Check sheet for the modelled part. Datum: model origin and axes. Units: mm. Coordinates: 2 decimals unless noted, no trailing zeros. Order: outer loops, then holes, each group sorted by start corner. A loop starts at its lowest first (then second) coordinate and runs counter-clockwise, first axis right, second up. Notation, with made-up numbers: (50, -35.5) -> (57, -35.5) arc R33 ccw to (57, -0.5) -> close; hole circle Ø1 at (79, 14). An arc over 180 degrees is marked (long way). Put each result on its own line as item: value. Start each with the question number.
```python
from build123d import *

# Parameters (mm, degrees)
F0_W      = 80
F0_H      = 120
F0_R      = 9.75
F0_R_2    = 4.25
F1_DEPTH  = 4
F3_W      = 80
F3_H      = 20
F4_DEPTH  = 10
F5_W      = 6
F5_H      = 6
F5_R      = 0.95
F6_DEPTH  = 10
F7_R      = 2.99999
F11_W     = 97.9346781969
F11_H     = 127.8536170721
F11_W_2   = 72.8027671576
F11_H_2   = 72.8027634323
F12_DEPTH = 10


# Not quite as in the source:
# - a fillet or chamfer is up to 0.001 mm smaller than in the source, because OpenCascade refuses the exact size


with BuildPart() as f1:
    # F0 (on Front) → F1 (new body)
    with BuildSketch(Plane.XZ):
        Rectangle(F0_W, F0_H)
        with Locations((0, -24.624)):
            Circle(F0_R, mode=Mode.SUBTRACT)
        with Locations((-24.032204955, 17.001)):
            Circle(F0_R, mode=Mode.SUBTRACT)
        with Locations((0, 3.126)):
            Circle(F0_R, mode=Mode.SUBTRACT)
        with Locations((0, 29.876)):
            Circle(F0_R_2, mode=Mode.SUBTRACT)
        with Locations((24.032204955, 17.001)):
            Circle(F0_R, mode=Mode.SUBTRACT)
    extrude(amount=F1_DEPTH)

    # F3 (on face) → F4 (cut)
    with BuildSketch(Plane.XZ.offset(4)):
        with Locations((0, -50)):
            Rectangle(F3_W, F3_H)
    extrude(amount=-F4_DEPTH, mode=Mode.SUBTRACT)

    # F8: F6 across plane


with BuildPart() as f6:
    # F5 (on face) → F6 (new body)
    with BuildSketch(Plane.XZ.offset(4)):
        with Locations((43, 3)):
            Rectangle(F5_W, F5_H)
        with Locations((42.5, 3.126)):
            Circle(F5_R, mode=Mode.SUBTRACT)
    extrude(amount=-F6_DEPTH)

    # F7 (radius 3 in the source; OpenCascade refuses exactly that, so slightly less here)
    f7_edges = [f6.edges().sort_by_distance(p)[0] for p in [
        (46, 1, 0),
        (46, 1, 6),
    ]]
    fillet(f7_edges, radius=F7_R)


with BuildPart() as f1_1:
    add(f1.part)
    add(f6.part.mirror(Plane.YZ))


with BuildPart() as f12_tool:
    # F11 (on face) → F12 (new body)
    with BuildSketch(Plane.XZ.offset(4)):
        with Locations((1.1506490409, -1.4746189117)):
            Rectangle(F11_W, F11_H)
        with Locations((0.1533515751, -0.2778600901)):
            Rectangle(F11_W_2, F11_H_2, mode=Mode.SUBTRACT)
    extrude(amount=-F12_DEPTH)


with BuildPart() as f1_2:
    add(f1_1.part)

    # F12: cut by f12_tool
    add(f12_tool.part, mode=Mode.SUBTRACT)


with BuildPart() as f6_1:
    add(f6.part)

    # F12: cut by f12_tool
    add(f12_tool.part, mode=Mode.SUBTRACT)


solid = f1_2.part
```
1) Sectioned sample at A-A (x = -28.5). Record the boundary of the cut face in (y, z), plus the area to 3 significant figures.
2) Sectioned sample at D-D (z = 10). Record the boundary of the cut face in (x, y).
3) Sectioned sample at B-B (x = 0). Record the boundary of the cut face in (y, z), plus the area to 3 significant figures.
4) Scan lines: line 1 along X through (y, z) = (-1.6, 14); line 2 along Z through (x, y) = (-5.5, -2.6); line 3 along X through (y, z) = (-2.25, 21). Record each from-to range of solid material in increasing order. Write a range as [from, to].
5) Mould release check, pull along Z, two halves, no side actions. Record for faces 1 (the flat face through (0, -2, 36.124)), 2 (the flat face through (0, -2, -36.679)), 3 (the cylindrical face through (-7.737, -1.972, -2.807)), 4 (the flat face through (1, -4, -8)): +Z half, -Z half, draft (parallel to the pull), parting line (faces both ways), or undercut.
6) Sectioned sample at C-C (y = -2.9). Record the boundary of the cut face in (x, z).
Entries:
1. outline: (-4, -36.68) -> (0, -36.68) -> (0, 8.33) -> (-4, 8.33) -> close; (-4, 25.67) -> (0, 25.67) -> (0, 36.12) -> (-4, 36.12) -> close
1. area: 222 mm2
2. outline: (-36.25, -4) -> (-30.82, -4) -> (-30.82, 0) -> (-36.25, 0) -> close; (-17.25, -4) -> (-6.91, -4) -> (-6.91, 0) -> (-17.25, 0) -> close; (6.91, -4) -> (17.25, -4) -> (17.25, 0) -> (6.91, 0) -> close; (30.82, -4) -> (36.55, -4) -> (36.55, 0) -> (30.82, 0) -> close
3. outline: (-4, -36.68) -> (0, -36.68) -> (0, -34.37) -> (-4, -34.37) -> close; (-4, -14.87) -> (0, -14.87) -> (0, -6.62) -> (-4, -6.62) -> close; (-4, 12.88) -> (0, 12.88) -> (0, 25.63) -> (-4, 25.63) -> close; (-4, 34.13) -> (0, 34.13) -> (0, 36.12) -> (-4, 36.12) -> close
3. area: 101 mm2
4. line 1: x = [-36.25, -33.31], [-14.76, 14.76], [33.31, 36.55]
4. line 2: z = [-36.68, -32.67], [-16.57, -4.92], [11.18, 36.12]
4. line 3: x = [-36.25, -32.92], [-15.14, 15.14], [32.92, 36.55]
5. face 1: +Z half
5. face 2: -Z half
5. face 3: undercut
5. face 4: draft
6. outline: (-36.25, -36.68) -> (36.55, -36.68) -> (36.55, 36.12) -> (-36.25, 36.12) -> close; hole circle Ø19.5 at (-24.03, 17); hole circle Ø19.5 at (0, -24.62); hole circle Ø19.5 at (0, 3.13); hole circle Ø8.5 at (0, 29.88); hole circle Ø19.5 at (24.03, 17)
